Input: dimensioned drawing with shaded views. Units: mm. Origin: part minimum x, y, z. Give positions to 0.01 mm unless a question says otherwise; leave off trailing zeros. Write each loop counter-clockwise with the first axis right and the second up, starting at its lowest first coordinate (ties: lowest second). Pieces come first, ordered by that corner, then holes.
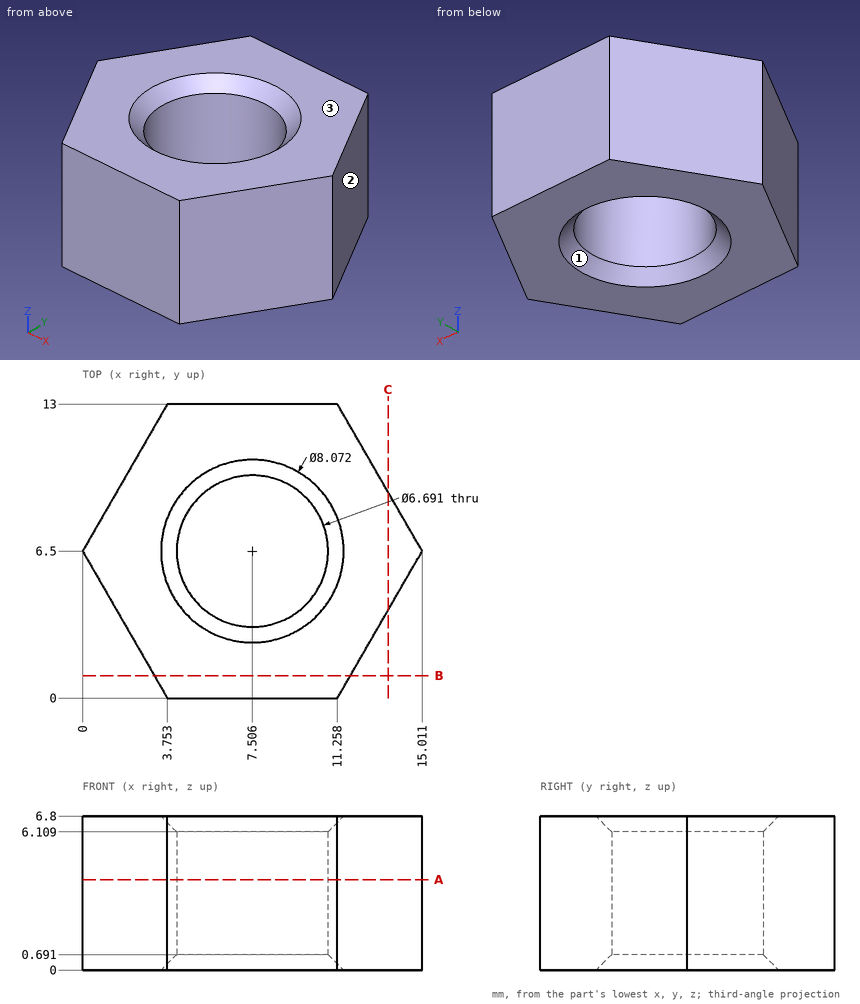
Item 1: Section A-A (z = 4). Return loops of the section in (x, y) (1 decimal).
Item 2: Mould query, pull axis X, two halves, no side actions, for the marked faces 1, 2 and 3. Classes: +X half, -X half, draft (parallel to the pull), parting line (faces both ways), or undercut.
Item 3: Section C-C (x = 13.5). Return loops of the section in (y, z).
Item 4: Ray query, line 1 (X direction, y = 9.5, z = 2.75) (1 decimal); line 2 (Y direction, x = 6.75, z = 4.5); line 3 (Y direction, x = 9.25, z = 3.75) (1 decimal). Return the intervals inside material, ascending.
Item 5: Section B-B (y = 1). Return loops of the section in (x, z) (1 decimal), and give its area (3 significant figures).
Solved:
1. outline: (0, 6.5) - (3.8, 0) - (11.3, 0) - (15, 6.5) - (11.3, 13) - (3.8, 13) - close; hole circle Ø6.7 at (7.5, 6.5)
2. face 1: undercut
2. face 2: +X half
2. face 3: draft
3. outline: (3.88, 0) - (9.12, 0) - (9.12, 6.8) - (3.88, 6.8) - close
4. line 1: x = 1.7 to 6, 9 to 13.3
4. line 2: y = 0 to 3.24, 9.76 to 13
4. line 3: y = 0 to 3.6, 9.4 to 13
5. outline: (3.2, 0) - (11.8, 0) - (11.8, 6.8) - (3.2, 6.8) - close
5. area: 58.9 mm2
